Check sheet for the modelled part. Datum: model origin and axes. Units: mm. Face numbers are marked on the shaded views. A direction names the side the tool comes from. Coordinates: 2 decimals unless noted, no trailing zeros. Write each loop counter-clockwise with the first axis right and the second up, starting at its lowest first coordinate (ties: lowest second). Pieces come first, ordered by that corner, then holes. Notation, with made-up numbers: (-4, 83.5) - (29, 83.5) arc R23 ccw to (29, 92.5) - close; hole circle Ø2 at (42, 26.25). An arc over 180 degrees is marked (long way). Use one line per item in the form item = value. Start each with the question number.
1. Draft check along Z on the marked faces 4, 5, 6 and 7. Enter one of: +Z half, -Z half, draft (parallel to the pull), parting line (faces both ways), or undercut.
2. Tool access check on the marked faces 1, 2 and 3. Record the directions out of +Z, -Z, +X, -X, +Y, -Y that give a thin tool (end or side, any length) a straight path to the whole face; none if there is none.
3. Cross-section at C-C on y = 0. Record the boundary of the cut face in (x, z).
4. Go/stop test with flat-tipped pins: pin 1 Ø1.2 at (x, z) = (0, 2.15) entering from -Y; pin 2 Ø1 at (x, z) = (1, -1.5) entering from -Y; pin 3 Ø2 at (x, y) = (0, 0) entering from +Z; pin 4 Ø1.5 at (y, z) = (-1.5, -2) entering from -X. Record where each tip stops, or that it passes through.
5. Cross-section at D-D on z = 3.75. Record the boundary of the cut face in (x, y).
6. Cross-section at A-A on x = -0.35. Record the boundary of the cut face in (y, z), then the cut area to 3 significant figures.
7. Cross-section at B-B on z = 2.15. Record the boundary of the cut face in (x, y), then the cut area to 3 significant figures.
8. Scan lines: line 1 along Y through (x, z) = (0, 3.5); line 2 along Z through (x, y) = (0, -1.75); line 3 along Z through (x, y) = (0.55, -1.1). Record each from-to range of solid material in increasing order.
```python
from build123d import *

# Parameters (mm, degrees)
SKETCH1_R           = 2.25
BOSS_EXTRUDE1_DEPTH = 6.15
SKETCH2_R           = 1
BOSS_EXTRUDE2_DEPTH = 5
SKETCH3_R           = 1.35
CUT_EXTRUDE1_DEPTH  = 6
SKETCH4_R           = 1
CUT_EXTRUDE2_DEPTH  = 6


with BuildPart() as part:
    # Sketch1 → Boss-Extrude1 (new body)
    with BuildSketch(Plane.XY):
        Circle(SKETCH1_R)
    extrude(amount=BOSS_EXTRUDE1_DEPTH)

    # Sketch2 → Boss-Extrude2 (add)
    with BuildSketch(Plane(origin=(0, 0, 0), x_dir=(-1, 0, 0), z_dir=(0, 0, -1))):
        Circle(SKETCH2_R)
    extrude(amount=BOSS_EXTRUDE2_DEPTH)

    # Sketch3 → Cut-Extrude1 (cut)
    with BuildSketch(Plane.XY.offset(6.15)):
        Circle(SKETCH3_R)
    extrude(amount=-CUT_EXTRUDE1_DEPTH, mode=Mode.SUBTRACT)

    # Sketch4 → Cut-Extrude2 (cut)
    with BuildSketch(Plane(origin=(0, -2.25, 0), x_dir=(-1, 0, 0), z_dir=(0, -1, 0))):
        with Locations(Location((0, -2.15, 0), (0, 0, 90))):
            Circle(SKETCH4_R)
    extrude(amount=-CUT_EXTRUDE2_DEPTH, mode=Mode.SUBTRACT)


solid = part.part
```
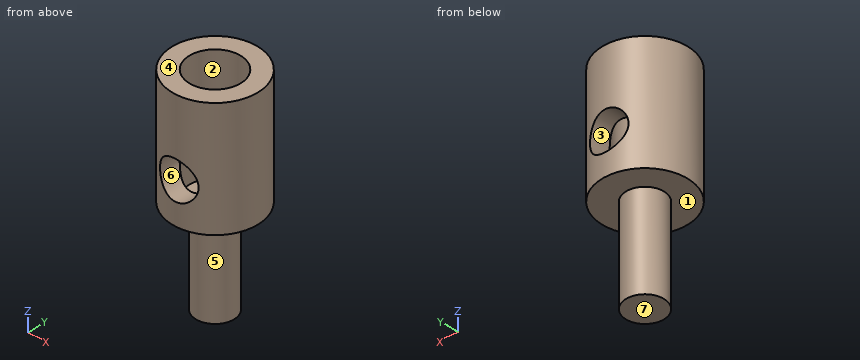
Final values:
q1.face_4 = +Z half
q1.face_5 = draft
q1.face_6 = undercut
q1.face_7 = -Z half
q2.face_1 = -Z
q2.face_2 = +Z
q2.face_3 = +Y, -Y
q3.outline = (-2.25, 0) - (-1, 0) - (-1, -5) - (1, -5) - (1, 0) - (2.25, 0) - (2.25, 6.15) - (1.35, 6.15) - (1.35, 0.15) - (-1.35, 0.15) - (-1.35, 6.15) - (-2.25, 6.15) - close
q4.pin_1 = through
q4.pin_2 = -0.87
q4.pin_3 = 0.15
q4.pin_4 = -0.66
q5.outline = circle Ø4.5 at (0, 0); hole circle Ø2.7 at (0, 0)
q6.outline = (-2.22, 0) - (-0.94, 0) - (-0.94, -5) - (0.94, -5) - (0.94, 0) - (2.22, 0) - (2.22, 1.21) - (1.3, 1.21) - (1.3, 0.15) - (-1.3, 0.15) - (-1.3, 1.21) - (-2.22, 1.21) - close; (-2.22, 3.09) - (-1.3, 3.09) - (-1.3, 6.15) - (-2.22, 6.15) - close; (1.3, 3.09) - (2.22, 3.09) - (2.22, 6.15) - (1.3, 6.15) - close
q6.area = 17.6 mm²
q7.outline = (-1, -2.02) - (-1, -0.91) arc R1.35 cw to (-1, 0.91) - (-1, 2.02) arc R2.25 ccw to start; (1, -2.02) arc R2.25 ccw to (1, 2.02) - (1, 0.91) arc R1.35 cw to (1, -0.91) - close
q7.area = 6.34 mm²
q8.line_1 = -2.25 to -1.35, 1.35 to 2.25
q8.line_2 = 0 to 1.15, 3.15 to 6.15
q8.line_3 = 0 to 0.15
